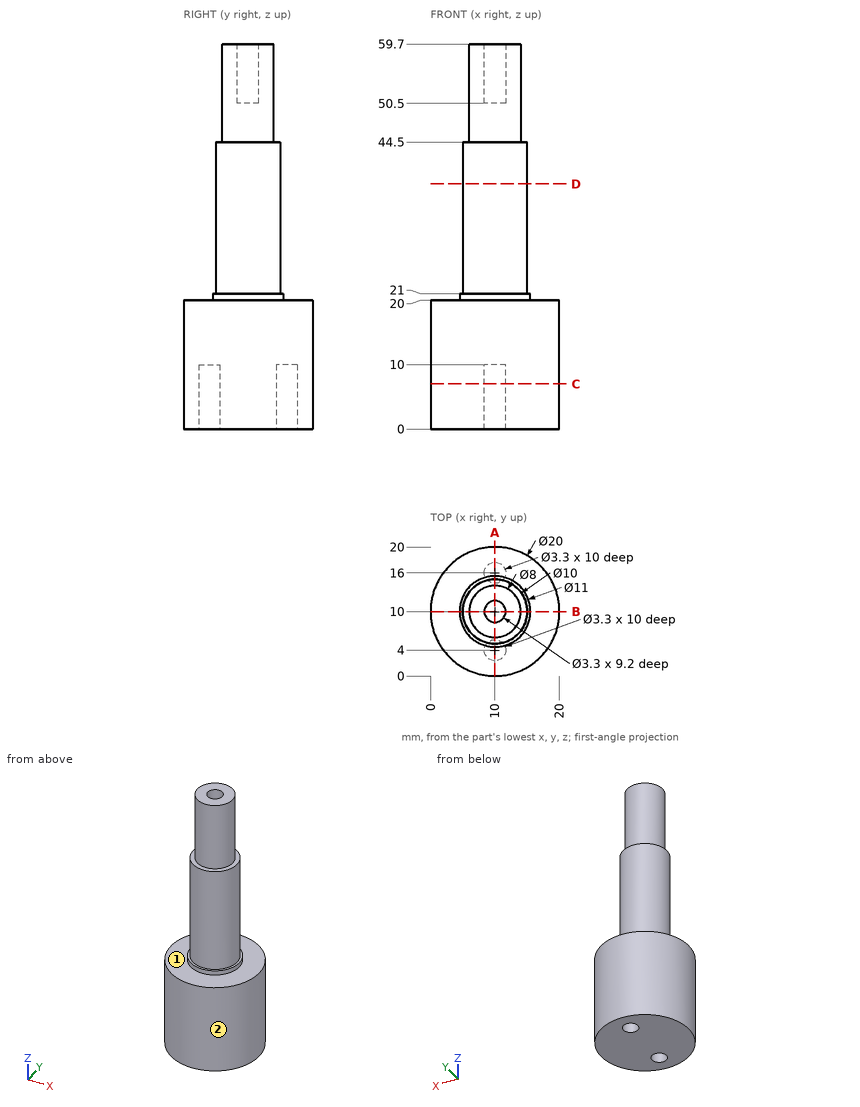
Geometry: see drawing. Coordinates: mm, zero at the bounding-box minimum. A direction names the side the tool comes from. Round coordinates to 2 decimals unless told otherwise and drop trailing zeros. Order: outer loops, then holes, each group sorted by start corner. A loop starts at its lowest first (then second) coordinate and runs counter-clockwise, first axis right, second up. Notation, with made-up numbers: (51, -1.5) -> (65, -1.5) arc R19 ccw to (65, 17.5) -> close; hole circle Ø9 at (24.25, 82). An arc over 180 degrees is marked (long way). Answer as CSV lines item,"result".
Item 1: Section B-B, the plane y = 10. Return loops of the section in (x, z).
A:
outline,"(0, 0) -> (20, 0) -> (20, 20) -> (15.5, 20) -> (15.5, 21) -> (15, 21) -> (15, 44.5) -> (14, 44.5) -> (14, 59.7) -> (11.65, 59.7) -> (11.65, 50.5) -> (8.35, 50.5) -> (8.35, 59.7) -> (6, 59.7) -> (6, 44.5) -> (5, 44.5) -> (5, 21) -> (4.5, 21) -> (4.5, 20) -> (0, 20) -> close"
Item 2: Reachability of the marked faces 1 and 2 from +Z, -Z, +X, -X, +Y, -Y: full face, straight path, thin tool, end or side. Return the list, or none.
A:
face 1,"+Z"
face 2,"+Z, -Z"
Item 3: Section C-C, the plane z = 7. Return loops of the section in (x, y), plus the area to 3 significant figures.
A:
outline,"circle Ø20 at (10, 10); hole circle Ø3.3 at (10, 4); hole circle Ø3.3 at (10, 16)"
area,"297 mm²"
Item 4: Section A-A, the plane x = 10. Return loops of the section in (y, z).
A:
outline,"(0, 0) -> (2.35, 0) -> (2.35, 10) -> (5.65, 10) -> (5.65, 0) -> (14.35, 0) -> (14.35, 10) -> (17.65, 10) -> (17.65, 0) -> (20, 0) -> (20, 20) -> (15.5, 20) -> (15.5, 21) -> (15, 21) -> (15, 44.5) -> (14, 44.5) -> (14, 59.7) -> (11.65, 59.7) -> (11.65, 50.5) -> (8.35, 50.5) -> (8.35, 59.7) -> (6, 59.7) -> (6, 44.5) -> (5, 44.5) -> (5, 21) -> (4.5, 21) -> (4.5, 20) -> (0, 20) -> close"
Item 5: Pin query (flat end, axial travel): pin 1 Ø2 at (x, z) = (7, 53.5) entering from -Y; pin 2 Ø6 at (y, z) = (4.5, 36.5) entering from -X; pin 3 Ø2.5 at (x, y) = (9.5, 16) entering from -Z; pin 4 Ø5 at (y, z) = (14, 47.5) entering from -X. Return the tip coordinate at first contact, or that it passes through.
A:
pin 1,"y = 6.54"
pin 2,"x = 5.67"
pin 3,"z = 0"
pin 4,"x = 6.29"
Item 6: Line query: L1, parallel to Y at x = 10, z = 5.5; L2, parallel to Y at x = 10, z = 53.5; L3, parallel to Z at x = 17.5, y = 7.75. Output: solid intervals per line, ascending.
A:
L1,"0 to 2.35, 5.65 to 14.35, 17.65 to 20"
L2,"6 to 8.35, 11.65 to 14"
L3,"0 to 20"
Item 7: Section D-D, the plane z = 38. Return loops of the section in (x, y), plus the area to 3 significant figures.
A:
outline,"circle Ø10 at (10, 10)"
area,"78.5 mm²"
